The drawing under review shows one solid part. Ordinate dimensions are in mm from its lowest x, y, z. Coordinates: 2 decimals unless noted, no trailing zeros. Order: outer loops, then holes, each group sorted by start corner. A loop starts at its lowest first (then second) coordinate and runs counter-clockwise, first axis right, second up. Notation, with made-up numbers: (31, 77) - (51, 77) arc R23 ccw to (51, 100) - close; hole circle Ø6 at (14, -40). An arc over 180 degrees is marked (long way). Write each question's results on one line, items separated by ' | '. Start each with the question number.
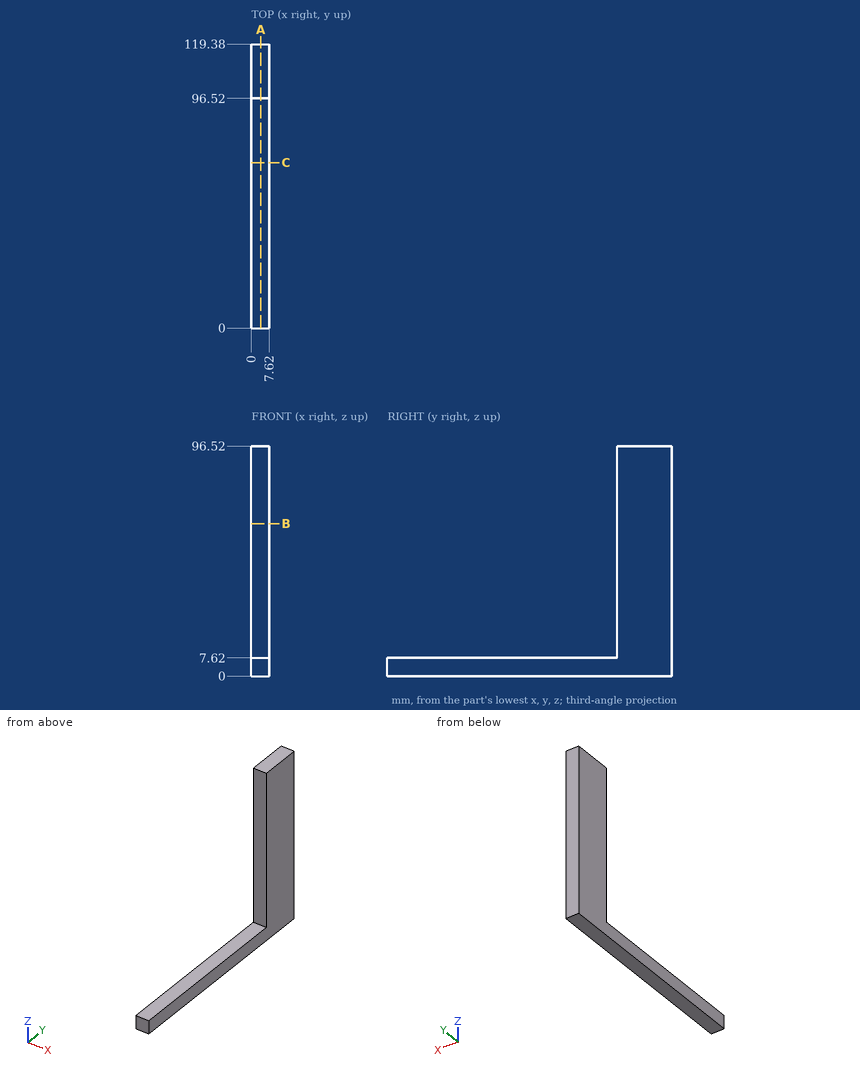
(1) Take a section at C-C (y = 69.5). State the section outline as (x, z) points.
(2) Take a section at A-A (x = 4). State the section outline as (y, z) points, plus the area to 3 significant figures.
(3) To check wall thickness, follow line 1 along Z through (x, y) = (1, 50); line 2 along Y through (x, z) = (6.5, 48). State the ranges of each line that lie inside material, in increasing order. Write a range as [from, to].
(4) Clearance check with flat-ended pins moving along their axes: pin 1 (3 mm diameter, centred on x = 4.5, y = 16.5, fed in from +Z); pin 2 (1.5 mm diameter, centred on x = 2, z = 23, fed in from -Y). State where each tip first meets the part, or that it passes through.
(5) Take a section at B-B (z = 64). State the section outline as (x, y) points.
Worked out:
1) outline: (0, 0) - (7.62, 0) - (7.62, 7.62) - (0, 7.62) - close
2) outline: (0, 0) - (119.38, 0) - (119.38, 96.52) - (96.52, 96.52) - (96.52, 7.62) - (0, 7.62) - close | area: 2,940 mm^2
3) line 1: [0, 7.62] | line 2: [96.52, 119.38]
4) pin 1: z = 7.62 | pin 2: y = 96.52
5) outline: (0, 96.52) - (7.62, 96.52) - (7.62, 119.38) - (0, 119.38) - close
